The listing builds one solid part. Answer for the finished solid, in the listing's coordinates (mm). Round coordinates to 2 decimals unless told otherwise and drop trailing zeros. Order: outer loops, then holes, each group sorted by start corner. A loop starts at its lowest first (then second) coordinate and runs counter-clockwise, first axis right, second up. Notation, with made-up numbers: (-33, 12.25) - (9, 12.25) arc R32 cw to (9, 39.25) - close; hole circle Ø8 at (-14, 87.5). An arc over 180 degrees is marked (long way). Write item = value, one per line.
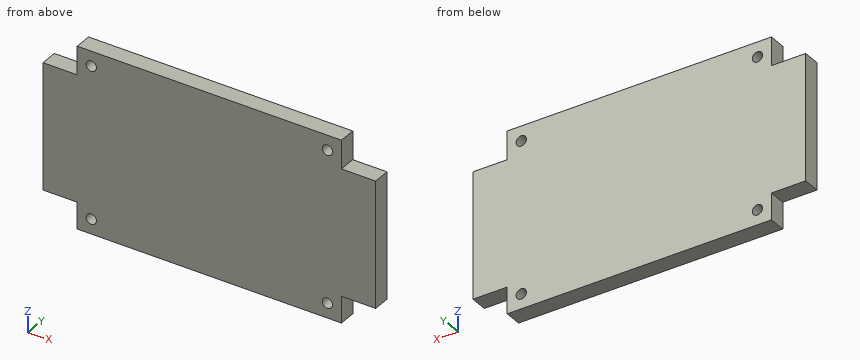
from build123d import *

# Parameters (mm, degrees)
SKETCH_1_W      = 77.14
SKETCH_1_H      = 52.9
SKETCH_1_R      = 1.5
EXTRUDE_1_DEPTH = 5
SKETCH_2_W      = 36.844868946
SKETCH_2_H      = 5
EXTRUDE_2_DEPTH = 10


with BuildPart() as part:
    # 草图1 → 凸台-拉伸1 (new body)
    with BuildSketch(Plane(origin=(0, 0, 0), x_dir=(1, 0, 0), z_dir=(0, 1, 0))):
        Rectangle(SKETCH_1_W, SKETCH_1_H)
        with Locations(Location((34.475, -22.13, 0), (0, 0, 270))):
            Circle(SKETCH_1_R, mode=Mode.SUBTRACT)
        with Locations(Location((34.475, 22.13, 0), (0, 0, 270))):
            Circle(SKETCH_1_R, mode=Mode.SUBTRACT)
        with Locations(Location((-34.475, 22.13, 0), (0, 0, 270))):
            Circle(SKETCH_1_R, mode=Mode.SUBTRACT)
        with Locations(Location((-34.475, -22.13, 0), (0, 0, 270))):
            Circle(SKETCH_1_R, mode=Mode.SUBTRACT)
    extrude(amount=EXTRUDE_1_DEPTH)

    # 草图2 → 凸台-拉伸2 (add)
    with BuildSketch(Plane.ZY.offset(38.57)):
        with Locations((-0.272252726, 2.5)):
            Rectangle(SKETCH_2_W, SKETCH_2_H)
    extrude_2 = extrude(amount=EXTRUDE_2_DEPTH)

    # 镜向1: 凸台-拉伸2 across plane
    add(extrude_2.mirror(Plane(origin=(0, 0, 0), x_dir=(0, 0, 1), z_dir=(1, 0, 0))))


solid = part.part
Q1. Find the intervals of material crossed by line 1 (X direction, y = 1.3, z = -22.13) (3 decimals); line 2 (X direction, y = 3.6, z = 22.5); line 3 (Z direction, x = 44.5, y = 0.2), in increasing order. Write a range as from..to.
Model answer:
line_1 = -38.57..-35.975, -32.975..32.975, 35.975..38.57
line_2 = -38.57..-35.93, -33.02..33.02, 35.93..38.57
line_3 = -18.69..18.15
Q2. Section A-A on z = 22.13 is taken. Determine the outline of the cut face in (x, y) (3 decimals), then the cut area to 3 significant figures.
Model answer:
outline = (-38.57, 0) - (-35.975, 0) - (-35.975, 5) - (-38.57, 5) - close; (-32.975, 0) - (32.975, 0) - (32.975, 5) - (-32.975, 5) - close; (35.975, 0) - (38.57, 0) - (38.57, 5) - (35.975, 5) - close
area = 356 mm^2
Q3. Flat-ended cylindrical pins translate along their axes: P1, Ø2.5, axis at x = -34.475, z = 22.13, coming from the -Y side; P2, Ø3.5, axis at x = 34.475, z = -22.13, coming from the +Y side; P3, Ø2.5, axis at y = 3.5, z = -24, coming from the +X side; P4, Ø1.5, axis at y = 2, z = 20.5, coming from the -X side. Find the tip coordinate at first contact, or state that the pin passes through.
Model answer:
P1 = through
P2 = 5
P3 = 38.57
P4 = -38.57
Q4. Section B-B on y = 3.8 is taken. Determine the outline of the cut face in (x, z) (3 decimals), then the cut area to 3 significant figures.
Model answer:
outline = (-48.57, -18.695) - (-38.57, -18.695) - (-38.57, -26.45) - (38.57, -26.45) - (38.57, -18.695) - (48.57, -18.695) - (48.57, 18.15) - (38.57, 18.15) - (38.57, 26.45) - (-38.57, 26.45) - (-38.57, 18.15) - (-48.57, 18.15) - close; hole circle Ø3 at (-34.475, -22.13); hole circle Ø3 at (-34.475, 22.13); hole circle Ø3 at (34.475, -22.13); hole circle Ø3 at (34.475, 22.13)
area = 4,790 mm^2
